Read the model definition and answer for the solid it produces. Units are mm, in the model's axes. Face numbers are marked on the shaded views. A direction names the side the tool comes from. Coordinates: 2 decimals unless noted, no trailing zeros. Write each loop counter-clockwise with the first axis right and the second up, starting at its lowest first coordinate (ties: lowest second). Pieces come first, ordered by that corner, then holes.
(1) Given pin 1 (2.5 mm diameter, centred on x = -1.5, z = 2.5, fed in from -Y); pin 2 (2.5 mm diameter, centred on x = 12, z = 1.5, fed in from -Y); pin 3 (1.5 mm diameter, centred on x = 1.5, z = 3, fed in from +Y), each flat-ended and moving along its own axis, determine where each tip first touches the part or whether it passes through.
(2) Determine the mould class of the marked faces 1, 2, 3 and 4 for opening direction Y: pulls with the +Y half, pulls with the -Y half, needs draft (parallel to the pull), parting line crosses it, or undercut.
(3) The part is cut by section C-C, the plane y = -19.5. Determine the outline of the cut face in (x, z).
(4) Straight lines are drawn through the part: line 1 along Y through (x, z) = (-0.5, 0.45); line 2 along X through (y, z) = (-6, 2.1); line 3 along X through (y, z) = (1.5, 2.85). For each, find the intervals that lie inside material, in ascending order.
(5) The part is cut by section A-A, the plane z = 3.6. State how many separate pieces and enclosed holes the cut face has, and give its area (3 significant figures).
(6) The part is cut by section B-B, the plane x = 7. Determine the outline of the cut face in (y, z).
(7) The part is cut by section D-D, the plane x = -8. Determine the outline of the cut face in (y, z).
(8) Which of the six approach directions +Z, -Z, +X, -X, +Y, -Y give full straight-line access (tool end or side, diameter ignored) to the marked faces 5 and 6?
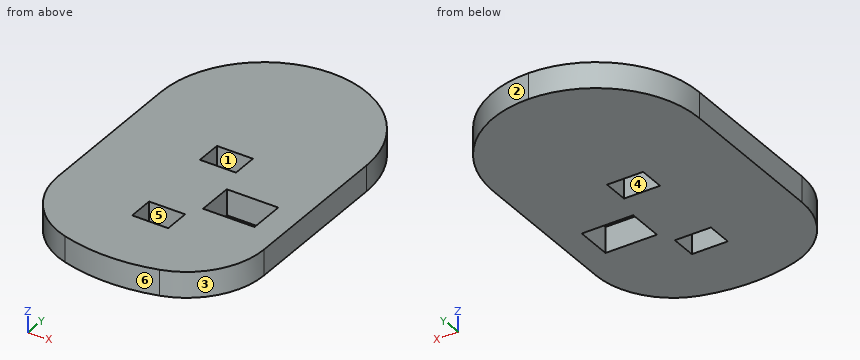
```python
from build123d import *

# Parameters (mm, degrees)
SKETCH1_R           = 33
BOSS_EXTRUDE1_DEPTH = 5
CUT_EXTRUDE3_START  = -10
CUT_EXTRUDE3_DEPTH  = 10
FILLET2_R           = 20
FILLET3_R           = 15
SKETCH11_W          = 7
SKETCH11_H          = 5
CUT_EXTRUDE4_DEPTH  = 10
SKETCH12_W          = 10
SKETCH12_H          = 7
CUT_EXTRUDE5_DEPTH  = 10


with BuildPart() as part:
    # Sketch1 → Boss-Extrude1 (new body)
    with BuildSketch(Plane.XY):
        Circle(SKETCH1_R)
    extrude(amount=BOSS_EXTRUDE1_DEPTH)

    # Sketch10 → Cut-Extrude3 (cut)
    with BuildSketch(Plane.XY.offset(5).offset(CUT_EXTRUDE3_START)):
        with BuildLine():
            Line((-20, 26.248809497), (-20, -26.248809497))
            ThreePointArc((-20, -26.248809497), (-33, 0), (-20, 26.248809497))
        make_face()
        with BuildLine():
            Line((20, 26.248809497), (20, -26.248809497))
            ThreePointArc((20, -26.248809497), (33, 0), (20, 26.248809497))
        make_face()
    extrude(amount=CUT_EXTRUDE3_DEPTH, mode=Mode.SUBTRACT)

    # Fillet2
    fillet2_edges = [part.edges().sort_by_distance(p)[0] for p in [
        (-20, 26.248809497, 2.5),
        (20, 26.248809497, 2.5),
    ]]
    fillet(fillet2_edges, radius=FILLET2_R - 0.0001)  # a hair under: the kernel refuses the full size

    # Fillet3
    fillet3_edges = [part.edges().sort_by_distance(p)[0] for p in [
        (-20, -26.248809497, 2.5),
        (20, -26.248809497, 2.5),
    ]]
    fillet(fillet3_edges, radius=FILLET3_R)

    # Sketch11 → Cut-Extrude4 (cut)
    with BuildSketch(Plane.XY.offset(5)):
        with Locations((0, 2)):
            Rectangle(SKETCH11_W, SKETCH11_H)
        with Locations((0, -18)):
            Rectangle(SKETCH11_W, SKETCH11_H)
    extrude(amount=-CUT_EXTRUDE4_DEPTH, mode=Mode.SUBTRACT)

    # Sketch12 → Cut-Extrude5 (cut)
    with BuildSketch(Plane.XY.offset(5)):
        with Locations((10, -9)):
            Rectangle(SKETCH12_W, SKETCH12_H)
    extrude(amount=-CUT_EXTRUDE5_DEPTH, mode=Mode.SUBTRACT)


solid = part.part
```
Computed:
1. pin 1: stops at y = -33
1. pin 2: stops at y = -31.15
1. pin 3: stops at y = 32.99
2. face 1: undercut
2. face 2: pulls with the +Y half
2. face 3: pulls with the -Y half
2. face 4: undercut
3. outline: (-19.84, 0) - (-3.5, 0) - (-3.5, 5) - (-19.84, 5) - close; (3.5, 0) - (19.84, 0) - (19.84, 5) - (3.5, 5) - close
4. line 1: y = -33 to -20.5, -15.5 to -0.5, 4.5 to 32.99
4. line 2: x = -20 to 5, 15 to 20
4. line 3: x = -20 to -3.5, 3.5 to 20
5. separate pieces: 1
5. enclosed holes: 3
5. area: 2,210 mm2
6. outline: (-32.25, 0) - (-12.5, 0) - (-12.5, 5) - (-32.25, 5) - close; (-5.5, 0) - (31.74, 0) - (31.74, 5) - (-5.5, 5) - close
7. outline: (-32.02, 0) - (31.33, 0) - (31.33, 5) - (-32.02, 5) - close
8. face 5: +Z, -Z
8. face 6: +Z, -Z, -Y
